CAD build for the part. Positions are in the model's coordinates, mm. A direction names the side the tool comes from. Round coordinates to 2 decimals unless told otherwise and drop trailing zeros. Order: outer loops, then holes, each group sorted by start corner. A loop starts at its lowest first (then second) coordinate and runs counter-clockwise, first axis right, second up. Notation, with made-up numbers: (58, -15) - (92, -15) arc R24 ccw to (92, 15) - close; hole circle Ø4 at (49, 62.5). An arc over 180 degrees is marked (long way). Write item = value, one per line.
from build123d import *

# Parameters (mm, degrees)
SKETCH1_R           = 12.5
BOSS_EXTRUDE1_DEPTH = 3
SKETCH2_R           = 4
SKETCH2_R_2         = 3
BOSS_EXTRUDE2_DEPTH = 10
SKETCH3_R           = 2.15
SKETCH3_R_2         = 3
CUT_EXTRUDE1_DEPTH  = 22.943108257
FILLET1_R           = 3


with BuildPart() as part:
    # Sketch1 → Boss-Extrude1 (new body)
    with BuildSketch(Plane(origin=(0, 0, 0), x_dir=(1, 0, 0), z_dir=(0, 1, 0))):
        with Locations(Location((0, 0, 0), (0, 0, 270))):
            Circle(SKETCH1_R)
    extrude(amount=BOSS_EXTRUDE1_DEPTH)

    # Sketch2 → Boss-Extrude2 (add)
    with BuildSketch(Plane(origin=(0, 3, 0), x_dir=(1, 0, 0), z_dir=(0, 1, 0))):
        with Locations(Location((4, 0, 0), (0, 0, 270))):
            Circle(SKETCH2_R)
        with Locations(Location((-4, 0, 0), (0, 0, 270))):
            Circle(SKETCH2_R_2)
    extrude(amount=BOSS_EXTRUDE2_DEPTH)

    # Sketch3 → Cut-Extrude1 (cut, through all)
    with BuildSketch(Plane(origin=(0, 13, 0), x_dir=(1, 0, 0), z_dir=(0, 1, 0))):
        with Locations(Location((-4, 0, 0), (0, 0, 270))):
            Circle(SKETCH3_R)
        with Locations(Location((4, 0, 0), (0, 0, 270))):
            Circle(SKETCH3_R_2)
    extrude(amount=-CUT_EXTRUDE1_DEPTH, mode=Mode.SUBTRACT)

    # Fillet1
    # the kernel refuses this fillet: 3 mm, written as the material it adds along each edge
    with BuildSketch(Plane(origin=(4, 3, 0), x_dir=(0, 0, 1), z_dir=(-1, 0, 0))) as fillet1_piece_1_section:
        with BuildLine():
            CenterArc((4 + FILLET1_R, FILLET1_R), FILLET1_R, 180, 90)
            Line((4, FILLET1_R), (4, 0))
            Line((4, 0), (4 + FILLET1_R, 0))
        make_face()
    fillet1_piece_1 = revolve(axis=Axis((4, 3, 0), (0, 1, 0)), mode=Mode.PRIVATE)
    fillet1_piece_1 = fillet1_piece_1 - Plane(origin=(-4, 3.851709764, 0), x_dir=(0, 0, 1), z_dir=(0, -1, 0)) * Cylinder(3, 29, mode=Mode.PRIVATE)
    add(fillet1_piece_1)
    with BuildSketch(Plane(origin=(-4, 3, 0), x_dir=(0, 0, 1), z_dir=(-1, 0, 0))) as fillet1_piece_2_section:
        with BuildLine():
            CenterArc((3 + FILLET1_R, FILLET1_R), FILLET1_R, 180, 90)
            Line((3, FILLET1_R), (3, 0))
            Line((3, 0), (3 + FILLET1_R, 0))
        make_face()
    fillet1_piece_2 = revolve(axis=Axis((-4, 3, 0), (0, 1, 0)), mode=Mode.PRIVATE)
    fillet1_piece_2 = fillet1_piece_2 - Plane(origin=(4, 3.853854746, 0), x_dir=(0, 0, 1), z_dir=(0, -1, 0)) * Cylinder(4, 24, mode=Mode.PRIVATE)
    add(fillet1_piece_2)


solid = part.part
(1) Band-saw the part on B-B on y = 10.75. List the corners of the cut face in (x, z).
Solved:
outline = circle Ø6 at (-4, 0); circle Ø8 at (4, 0); hole circle Ø4.3 at (-4, 0); hole circle Ø6 at (4, 0)
(2) Drop flat-ended pins along their axis: pin 1 (2 mm diameter, centred on y = 4.5, z = -2, fed in from -X); pin 2 (12 mm diameter, centred on x = 5, z = -4.5, fed in from -Y); pin 3 (6 mm diameter, centred on y = 8, z = 1.5, fed in from +X); pin 4 (3 mm diameter, centred on x = -5.5, y = 5, fed in from +Z). Give the stop position or say it passes through.
Solved:
pin_1 = -7.92
pin_2 = 0
pin_3 = 8.09
pin_4 = 4.13
(3) Band-saw the part on A-A on x = 4. List the corners of the cut face in (y, z), plus the area to 3 significant figures.
Solved:
outline = (0, -11.84) - (3, -11.84) - (3, -7) arc R3 cw to (6, -4) - (13, -4) - (13, -3) - (0, -3) - close; (0, 3) - (13, 3) - (13, 4) - (6, 4) arc R3 cw to (3, 7) - (3, 11.84) - (0, 11.84) - close
area = 76.9 mm²
(4) Probe line 1 along X through (y, z) = (6.75, 0); line 2 along X through (y, z) = (3.5, 0); line 3 along X through (y, z) = (1.25, 1). List the from-to ranges inside material, lowest first.
Solved:
line_1 = -7 to -6.15, -1.85 to -1, 0 to 1, 7 to 8
line_2 = -8.34 to -6.15, -1.85 to 1, 7 to 9.34
line_3 = -12.46 to -5.9, -2.1 to 1.17, 6.83 to 12.46
(5) Pull direction Z, two halves, no side cores. Call faces 1 (the cylindrical face through (-1.87, 6.59, -0.28)), 2 (the flat face through (0, 3, 8)), 3 (the cylindrical face through (0.095, 9.451, -0.867)): released by +Z, released by -Z, zero draft, split by the parting line, or undercut.
Solved:
face_1 = undercut
face_2 = zero draft
face_3 = split by the parting line
(6) Tool access for faces 4 (the cylindrical face through (-6.662, 9.451, 1.384)), 5 (the cylindrical face through (1.338, 6.591, 1.384)): list every direction of +Z, -Z, +X, -X, +Y, -Y with a clear straight run to the whole face (end or side of a thin tool).
Solved:
face_4 = +Y
face_5 = +Y, -Y
(7) Band-saw the part on C-C on z = 0. List the corners of the cut face in (x, y).
Solved:
outline = (-12.5, 0) - (-6.15, 0) - (-6.15, 13) - (-7, 13) - (-7, 6) arc R3 cw to (-10, 3) - (-12.5, 3) - close; (-1.85, 0) - (1, 0) - (1, 13) - (0, 13) - (0, 6) arc R3 cw to (-0.5, 4.34) arc R3 cw to (-1, 6) - (-1, 13) - (-1.85, 13) - close; (7, 0) - (12.5, 0) - (12.5, 3) - (11, 3) arc R3 cw to (8, 6) - (8, 13) - (7, 13) - close
(8) Band-saw the part on D-D on y = 2. List the corners of the cut face in (x, z), plus the area to 3 significant figures.
Solved:
outline = circle Ø25 at (0, 0); hole circle Ø4.3 at (-4, 0); hole circle Ø6 at (4, 0)
area = 448 mm²
